from build123d import *

# Parameters (mm, degrees)
SKETCH3_W               = 114.3
SKETCH3_H               = 19.05
BOSS_EXTRUDE1_DEPTH     = 3.81
BOSS_EXTRUDE2_START     = -22.225
BOSS_EXTRUDE2_OUTLINE_R = 13.5453125
BOSS_EXTRUDE2_DEPTH     = 44.45
SKETCH6_R               = 2.749999961
CUT_EXTRUDE5_DEPTH      = 7.62
CUT_EXTRUDE7_REACH      = 208.672
SKETCH7_RX              = 2.749999961
SKETCH7_RY              = 2.656295985
CUT_EXTRUDE8_REACH      = 221.372
CUT_EXTRUDE8_START      = -12.7
CUT_EXTRUDE9_REACH      = 237.378
SKETCH14_W              = 2
SKETCH14_H              = 6.499999954
MIRROR2_COPY_1_REACH    = 237.378
MIRROR2_COPY_1_SKETCH_W = 2
MIRROR2_COPY_1_SKETCH_H = 6.499999954
FILLET1_R               = 1.905


# Read off the part's stored shape, not the designer's step: Boss-Extrude2
with BuildPart() as part:
    # Sketch3 → Boss-Extrude1 (new body)
    with BuildSketch(Plane(origin=(0, 0, 0), x_dir=(1, 0, 0), z_dir=(0, 1, 0))):
        Rectangle(SKETCH3_W, SKETCH3_H)
    extrude(amount=BOSS_EXTRUDE1_DEPTH)

    # Boss-Extrude2 outline → Boss-Extrude2 (add)
    with BuildSketch(Plane.XY.offset(BOSS_EXTRUDE2_START)):
        with BuildLine():
            ThreePointArc((48.050005342, 31.090690807), (42.090813056, 22.523397373), (42.122274879, 12.087425946))
            ThreePointArc((42.122274879, 12.087425946), (41.198342199, 6.412778013), (36.071859255, 3.81))
            Line((36.071859255, 3.81), (-36.071859255, 3.81))
            ThreePointArc((-36.071859255, 3.81), (-41.198342199, 6.412778013), (-42.122274879, 12.087425946))
            ThreePointArc((-42.122274879, 12.087425946), (-49.981131055, 32.385454016), (-71.489167098, 29.042409074))
            ThreePointArc((-71.489167098, 29.042409074), (-76.865522705, 27.00523428), (-81.682836057, 30.143509735))
            Line((-81.682836057, 30.143509735), (-117.754695312, 92.621802688))
            ThreePointArc((-117.754695312, 92.621802688), (-118.063864905, 98.362856156), (-113.611441977, 102.000329294))
            ThreePointArc((-113.611441977, 102.000329294), (-104.557894696, 107.19106827), (-100.117997084, 116.635526893))
            Line((-100.117997084, 116.635526893), (-93.370404601, 117.225864741))
            Line((-93.370404601, 117.225864741), (-93.702467981, 121.021366541))
            Line((-93.702467981, 121.021366541), (-103.823806114, 120.135864194))
            ThreePointArc((-103.823806114, 120.135864194), (-130.235968745, 114.8821584), (-105.586989883, 125.727968673))
            Line((-105.586989883, 125.727968673), (-96.78817178, 130.807968673))
            Line((-96.78817178, 130.807968673), (-98.69317178, 134.107525461))
            Line((-98.69317178, 134.107525461), (-104.559079836, 130.720841866))
            ThreePointArc((-104.559079836, 130.720841866), (-127.602080191, 132.935148506), (-132.347716126, 110.277656173))
            Line((-132.347716126, 110.277656173), (-53.749017487, -25.859283278))
            ThreePointArc((-53.749017487, -25.859283278), (-50.679795969, -28.55091831), (-46.606255237, -28.817912275))
            Line((-46.606255237, -28.817912275), (63.150672714, 0.591367933))
            ThreePointArc((63.150672714, 0.591367933), (76.010547273, 17.706450636), (62.468787305, 34.28725781))
            Line((62.468787305, 34.28725781), (62.468787305, 41.060625))
            Line((62.468787305, 41.060625), (58.658787305, 41.060625))
            Line((58.658787305, 41.060625), (58.658787305, 30.900625))
            ThreePointArc((58.658787305, 30.900625), (61.590529512, 4.131077991), (52.934290882, 29.631534697))
            Line((52.934290882, 29.631534697), (48.640489342, 38.839621813))
            Line((48.640489342, 38.839621813), (45.187456674, 37.229446236))
            Line((45.187456674, 37.229446236), (48.050005342, 31.090690807))
        make_face()
        with Locations((-58.658787305, 17.3553125)):
            Circle(BOSS_EXTRUDE2_OUTLINE_R, mode=Mode.SUBTRACT)
    extrude(amount=BOSS_EXTRUDE2_DEPTH)

    # Sketch6 → Cut-Extrude5 (cut)
    with BuildSketch(Plane(origin=(-48.209604448, -27.833828106, 0), x_dir=(0, 0, -1), z_dir=(0.8660254037844433, 0.4999999999999923, 0))):
        with Locations(Location((-10.795, 85.238322473, 0), (0, 0, 90))):
            Circle(SKETCH6_R)
        with Locations(Location((10.795, 85.238322473, 0), (0, 0, 90))):
            Circle(SKETCH6_R)
    extrude(amount=-CUT_EXTRUDE5_DEPTH, mode=Mode.SUBTRACT)

    # Cut-Extrude7: up to this plane
    cut_extrude7_end = Plane(origin=(0, 3.81, 0), z_dir=(0, -1, 0))
    # Sketch7 → Cut-Extrude7 (cut, up to the surface)
    with BuildSketch(Plane(origin=(4.082450956, -15.235914386, 0), x_dir=(0.9659258262890681, 0.25881904510252174, 0), z_dir=(0.25881904510252174, -0.9659258262890681, 0)), mode=Mode.PRIVATE) as cut_extrude7_sk1:
        with Locations(Location((4.66627796, 0), (0, 0, -90))):
            Ellipse(SKETCH7_RX, SKETCH7_RY)
    cut_extrude7_tool1 = split(extrude(cut_extrude7_sk1.sketch, amount=-CUT_EXTRUDE7_REACH, mode=Mode.PRIVATE), bisect_by=cut_extrude7_end, keep=Keep.BOTH, mode=Mode.PRIVATE)
    add(cut_extrude7_tool1.solids().sort_by_distance((8.589729, -14.028193, 0))[0], mode=Mode.SUBTRACT)
    # Sketch7 → Cut-Extrude7 (cut, up to the surface)
    with BuildSketch(Plane(origin=(4.082450956, -15.235914386, 0), x_dir=(0.9659258262890681, 0.25881904510252174, 0), z_dir=(0.25881904510252174, -0.9659258262890681, 0)), mode=Mode.PRIVATE) as cut_extrude7_sk2:
        with Locations(Location((-16.18806063, 0), (0, 0, -90))):
            Ellipse(SKETCH7_RX, SKETCH7_RY)
    cut_extrude7_tool2 = split(extrude(cut_extrude7_sk2.sketch, amount=-CUT_EXTRUDE7_REACH, mode=Mode.PRIVATE), bisect_by=cut_extrude7_end, keep=Keep.BOTH, mode=Mode.PRIVATE)
    add(cut_extrude7_tool2.solids().sort_by_distance((-11.554015, -19.425693, 0))[0], mode=Mode.SUBTRACT)

    # Cut-Extrude8: up to this plane
    cut_extrude8_end = Plane(origin=(0, 3.81, 0), z_dir=(0, -1, 0))
    # Sketch11 → Cut-Extrude8 (cut, up to the surface)
    with BuildSketch(Plane(origin=(4.082450956, -15.235914386, 0), x_dir=(0.9659258262890681, 0.25881904510252174, 0), z_dir=(0.25881904510252174, -0.9659258262890681, 0)).offset(CUT_EXTRUDE8_START), mode=Mode.PRIVATE) as cut_extrude8_sk1:
        Polygon((-11.453788359, 0), (-13.820924494, 4.100000055), (-18.555196765, 4.100000055), (-20.9223329, 0), (-18.555196765, -4.100000055), (-13.820924494, -4.100000055), align=None)
    cut_extrude8_tool1 = split(extrude(cut_extrude8_sk1.sketch, amount=-CUT_EXTRUDE8_REACH, mode=Mode.PRIVATE), bisect_by=cut_extrude8_end, keep=Keep.BOTH, mode=Mode.PRIVATE)
    add(cut_extrude8_tool1.solids().sort_by_distance((-14.841017, -7.158435, 0))[0], mode=Mode.SUBTRACT)
    # Sketch11 → Cut-Extrude8 (cut, up to the surface)
    with BuildSketch(Plane(origin=(4.082450956, -15.235914386, 0), x_dir=(0.9659258262890681, 0.25881904510252174, 0), z_dir=(0.25881904510252174, -0.9659258262890681, 0)).offset(CUT_EXTRUDE8_START), mode=Mode.PRIVATE) as cut_extrude8_sk2:
        Polygon((9.400550231, 0), (7.033414095, 4.100000055), (2.299141825, 4.100000055), (-0.067994311, 0), (2.299141825, -4.100000055), (7.033414095, -4.100000055), align=None)
    cut_extrude8_tool2 = split(extrude(cut_extrude8_sk2.sketch, amount=-CUT_EXTRUDE8_REACH, mode=Mode.PRIVATE), bisect_by=cut_extrude8_end, keep=Keep.BOTH, mode=Mode.PRIVATE)
    add(cut_extrude8_tool2.solids().sort_by_distance((5.302727, -1.760935, 0))[0], mode=Mode.SUBTRACT)

    # Sketch14 → Cut-Extrude9 (cut, up to next)
    with BuildSketch(Plane(origin=(-82.743554889, 143.316041067, 0), x_dir=(0.8660254037844421, 0.499999999999994, 0), z_dir=(-0.499999999999994, 0.8660254037844421, 0)), mode=Mode.PRIVATE) as cut_extrude9_sk1:
        with Locations((-21.803714806, 0)):
            Rectangle(SKETCH14_W, SKETCH14_H)
    cut_extrude9_tool1 = extrude(cut_extrude9_sk1.sketch, amount=-CUT_EXTRUDE9_REACH, mode=Mode.PRIVATE) & part.part
    cut_extrude9 = cut_extrude9_tool1.solids().sort_by_distance((-101.626126, 132.414184, 0))[0]
    add(cut_extrude9, mode=Mode.SUBTRACT)

    # Mirror1: Cut-Extrude9 across plane
    add(cut_extrude9.mirror(Plane(origin=(-44.723303861, 141.844198069, 0), x_dir=(0, 0, 1), z_dir=(0.30070579950426285, -0.9537169507482302, 0))), mode=Mode.SUBTRACT)

    # Mirror2: Cut-Extrude9 across plane
    add(cut_extrude9.mirror(Plane(origin=(-51.509161237, 29.738828106, 0), x_dir=(0, 0, 1), z_dir=(0.8660254037844365, -0.500000000000004, 0))), mode=Mode.SUBTRACT)

    # Mirror2 copy 1 sketch → Mirror2 copy 1 (cut, up to next)
    with BuildSketch(Plane(origin=(37.404082957, 53.920945037, 0), x_dir=(-0.42261826174070477, 0.9063077870366477, 0), z_dir=(-0.9063077870366478, -0.42261826174070427, 0)), mode=Mode.PRIVATE) as mirror2_copy_1_sk1:
        with Locations((-21.803714806, 0)):
            Rectangle(MIRROR2_COPY_1_SKETCH_W, MIRROR2_COPY_1_SKETCH_H)
    mirror2_copy_1_tool1 = extrude(mirror2_copy_1_sk1.sketch, amount=-MIRROR2_COPY_1_REACH, mode=Mode.PRIVATE) & part.part
    add(mirror2_copy_1_tool1.solids().sort_by_distance((46.618730656, 34.16006836, 0))[0], mode=Mode.SUBTRACT)

    # Fillet1
    fillet1_edges = [part.edges().sort_by_distance(p)[0] for p in [
        (-105.586989883, 125.727968673, 0),
        (-103.823806114, 120.135864194, 0),
        (-100.117997084, 116.635526893, 0),
        (-104.559079836, 130.720841866, 0),
        (52.934290882, 29.631534697, 0),
        (58.658787305, 30.900625, 0),
        (48.050005342, 31.090690807, 0),
        (62.468787305, 34.28725781, 0),
        (62.468787305, 41.060625, 0),
        (45.187456674, 37.229446236, 0),
        (48.640489342, 38.839621813, 0),
        (58.658787305, 41.060625, 0),
        (-93.370404601, 117.225864741, 0),
        (-93.702467981, 121.021366541, 0),
        (-96.78817178, 130.807968673, 0),
        (-98.69317178, 134.107525461, 0),
    ]]
    fillet(fillet1_edges, radius=FILLET1_R - 0.0001)  # a hair under: the kernel refuses the full size


solid = part.part
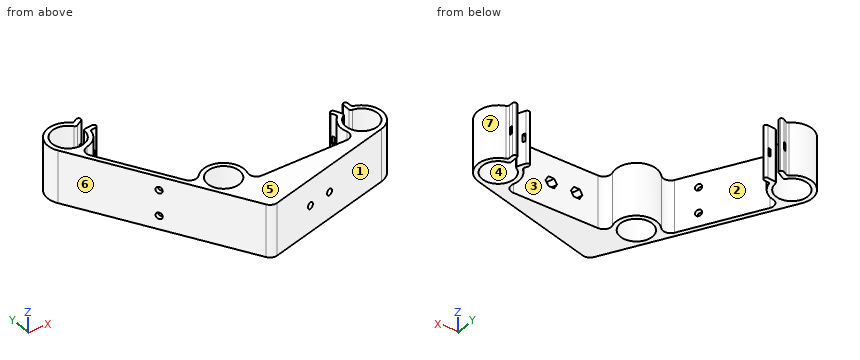
CAD build for the part. Positions are in the model's coordinates, mm. Face numbers are marked on the shaded views. A direction names the side the tool comes from. Round coordinates to 2 decimals unless told otherwise and drop trailing zeros. Loops run counter-clockwise (first coordinate to the right, second up) from the corner with the lowest first, then second, coordinate; pieces in that order, holes last.
(1) Which spindle directions (+Z, -Z, +X, -X, +Y, -Y) get a long thin tool onto all of the face, cutting with end or side? Do the marked faces 1, 2 and 3. Say none if no direction does.
(2) Drop flat-ended pins along their axis: pin 1 (10 mm diameter, centred on y = 76, z = -0.5, fed in from -X); pin 2 (1.5 mm diameter, centred on x = 54, z = 17, fed in from +Y); pin 3 (4 mm diameter, centred on x = 16.5, z = -15, fed in from -Y). Give the stop position or say it passes through.
(3) Two-plate mould, pull along X, no slides. Class the marked faces 4, 5, 6 and 7: +X half, -X half, draft (parallel to the pull), parting line (faces both ways), or undercut.
(4) Cut at A-A (x = -69). Give the cut face in (y, z) (3 decimals).
(5) Wall check: line 1 along Y through (x, z) = (-102, 15); line 2 along X through (y, z) = (6, -12); line 3 along X through (y, z) = (21, 3.5). Give the ranges that are in metal, low to high.
Findings below:
1. face 1: +Z, -Z, +X, -Y
1. face 2: +Z, -Z
1. face 3: +Z, -Z, +Y
2. pin 1: stops at x = -115.44
2. pin 2: stops at y = 4.94
2. pin 3: stops at y = -12.44
3. face 4: undercut
3. face 5: draft
3. face 6: -X half
3. face 7: +X half
4. outline: (0.556, -22.225) - (8.607, -22.225) - (8.607, 22.225) - (0.556, 22.225) - close; (26.104, -22.225) - (31.293, -22.225) - (31.293, 22.225) - (26.104, 22.225) - close
5. line 1: y = 57.71 to 65.33, 110.8 to 120.3, 127.8 to 132.2
5. line 2: x = -72.14 to -66.04, -51.27 to -40.87, 40.87 to 51.27, 66.04 to 71.78
5. line 3: x = -80.8 to -71.7, -45.61 to -41.69, 41.69 to 45.61, 71.7 to 75.63
